```python
from build123d import *

# Parameters (mm, degrees)
TOP_EDGE_OUTLINE_W   = 86.5
TOP_EDGE_OUTLINE_H   = 39.5
TOP_EDGE_DEPTH       = 3
TOP_EDGE_DRAFT       = 45
SKETCH13_W           = 72
SKETCH13_H           = 25
DISPLAY_HOLE_DEPTH   = 6
SKETCH14_W           = 92.5
SKETCH14_H           = 45.5
SKETCH14_W_2         = 89.5
SKETCH14_H_2         = 42.5
BOSS_EXTRUDE5_DEPTH  = 5
SKETCH15_W           = 128.5
SKETCH15_H           = 45.5
SKETCH15_W_2         = 89.5
SKETCH15_H_2         = 42.5
BOSS_EXTRUDE6_DEPTH  = 2
SKETCH16_W           = 128.5
SKETCH16_H           = 45.5
SKETCH16_W_2         = 125.5
SKETCH16_H_2         = 42.5
BOSS_EXTRUDE7_DEPTH  = 37
LOFT2_OUTLINE_W      = 33
LOFT2_OUTLINE_H      = 42.5
LOFT2_DEPTH          = 1.5
LOFT2_DRAFT          = 45
SKETCH19_R           = 2.75
SKETCH19_R_2         = 2
BOSS_EXTRUDE8_DEPTH  = 1
CUT_EXTRUDE3_START   = -11
SKETCH20_R           = 2
CUT_EXTRUDE3_DEPTH   = 11
SKETCH21_W           = 12
SKETCH21_H           = 8
CUT_EXTRUDE4_DEPTH   = 11
SKETCH22_W           = 4
SKETCH22_H           = 15
BOSS_EXTRUDE9_DEPTH  = 3
SKETCH24_W           = 42.5
SKETCH24_H           = 37
CUT_EXTRUDE5_DEPTH   = 17
SKETCH26_W           = 65.330388672
SKETCH26_H           = 66.528532866
CUT_EXTRUDE6_DEPTH   = 47
SKETCH27_W           = 135.174847233
SKETCH27_H           = 89.815373094
CUT_EXTRUDE7_DEPTH   = 47
SKETCH28_W           = 107.897480511
SKETCH28_H           = 56.576939502
SKETCH28_W_2         = 83.398406197
SKETCH28_H_2         = 34.654132256
CUT_EXTRUDE9_DEPTH   = 20.5
SKETCH29_W           = 89.2
SKETCH29_H           = 42.2
SKETCH29_W_2         = 86.2
SKETCH29_H_2         = 39.2
BOSS_EXTRUDE11_DEPTH = 5


# Read off the part's stored shape, not the designer's step: Top Edge, Loft2
with BuildPart() as part:
    # Top Edge outline → Top Edge (with draft: the straight prism first)
    with BuildSketch(Plane(origin=(0, 0, 0), x_dir=(1, 0, 0), z_dir=(0, 1, 0))):
        with Locations((0.25, -0.25)):
            Rectangle(TOP_EDGE_OUTLINE_W, TOP_EDGE_OUTLINE_H)
    extrude(amount=-TOP_EDGE_DEPTH)
    # Top Edge: the draft: its side faces are tilted about the plane it starts from
    top_edge_sides = [part.faces().sort_by_distance(p)[0] for p in [
        (-43, -1.5, 0.25),
        (0.25, -1.5, 20),
        (43.5, -1.5, 0.25),
        (0.25, -1.5, -19.5),
    ]]
    draft(top_edge_sides, Plane(origin=(0, 0, 0), x_dir=(1, 0, 0), z_dir=(0, 1, 0)), TOP_EDGE_DRAFT)

    # Sketch13 → Display Hole (cut)
    with BuildSketch(Plane(origin=(0, 0, 0), x_dir=(1, 0, 0), z_dir=(0, 1, 0))):
        Rectangle(SKETCH13_W, SKETCH13_H)
    extrude(amount=-DISPLAY_HOLE_DEPTH, mode=Mode.SUBTRACT)

    # Sketch14 → Boss-Extrude5 (add)
    with BuildSketch(Plane.XZ.offset(3)):
        with Locations((0.25, 0.25)):
            Rectangle(SKETCH14_W, SKETCH14_H)
        with Locations((0.25, 0.25)):
            Rectangle(SKETCH14_W_2, SKETCH14_H_2, mode=Mode.SUBTRACT)
    extrude(amount=BOSS_EXTRUDE5_DEPTH)

    # Sketch15 → Boss-Extrude6 (add)
    with BuildSketch(Plane.XZ.offset(8)):
        with Locations((18.25, 0.25)):
            Rectangle(SKETCH15_W, SKETCH15_H)
        with Locations((0.25, 0.25)):
            Rectangle(SKETCH15_W_2, SKETCH15_H_2, mode=Mode.SUBTRACT)
    extrude(amount=BOSS_EXTRUDE6_DEPTH)

    # Sketch16 → Boss-Extrude7 (add)
    with BuildSketch(Plane.XZ.offset(10)):
        with Locations((18.25, 0.25)):
            Rectangle(SKETCH16_W, SKETCH16_H)
        with Locations((18.25, 0.25)):
            Rectangle(SKETCH16_W_2, SKETCH16_H_2, mode=Mode.SUBTRACT)
    extrude(amount=BOSS_EXTRUDE7_DEPTH)


with BuildPart() as loft2_tool:
    # Loft2 outline → Loft2 (with draft: the straight prism first)
    with BuildSketch(Plane(origin=(0, -6.5, 0), x_dir=(1, 0, 0), z_dir=(0, 1, 0))):
        with Locations((64.5, -0.25)):
            Rectangle(LOFT2_OUTLINE_W, LOFT2_OUTLINE_H)
    extrude(amount=-LOFT2_DEPTH)
    # Loft2: the draft: its side faces are tilted about the plane it starts from
    loft2_sides = [loft2_tool.faces().sort_by_distance(p)[0] for p in [
        (81, -7.25, 0.25),
        (64.5, -7.25, -21),
        (48, -7.25, 0.25),
        (64.5, -7.25, 21.5),
    ]]
    draft(loft2_sides, Plane(origin=(0, -6.5, 0), x_dir=(1, 0, 0), z_dir=(0, 1, 0)), LOFT2_DRAFT)


with BuildPart() as part_1:
    add(part.part)

    # Loft2: add loft2_tool
    add(loft2_tool.part)

    # Sketch19 → Boss-Extrude8 (add)
    with BuildSketch(Plane(origin=(0, -6.5, 0), x_dir=(1, 0, 0), z_dir=(0, 1, 0))):
        with Locations(Location((64.5, 3, 0), (0, 0, 270))):
            Circle(SKETCH19_R)
        with Locations(Location((64.5, 3, 0), (0, 0, 270))):
            Circle(SKETCH19_R_2, mode=Mode.SUBTRACT)
    extrude(amount=BOSS_EXTRUDE8_DEPTH)

    # Sketch20 → Cut-Extrude3 (cut)
    with BuildSketch(Plane(origin=(0, -6.5, 0), x_dir=(1, 0, 0), z_dir=(0, 1, 0)).offset(CUT_EXTRUDE3_START)):
        with Locations(Location((64.5, 3, 0), (0, 0, 90))):
            Circle(SKETCH20_R)
    extrude(amount=CUT_EXTRUDE3_DEPTH, mode=Mode.SUBTRACT)

    # Sketch21 → Cut-Extrude4 (cut)
    with BuildSketch(Plane(origin=(82.5, 0, 0), x_dir=(0, 0, -1), z_dir=(1, 0, 0))):
        with Locations((0, -43)):
            Rectangle(SKETCH21_W, SKETCH21_H)
    extrude(amount=-CUT_EXTRUDE4_DEPTH, mode=Mode.SUBTRACT)

    # Sketch22 → Boss-Extrude9 (add)
    with BuildSketch(Plane.XZ.offset(3)):
        with Locations((-38, 0)):
            Rectangle(SKETCH22_W, SKETCH22_H)
    extrude(amount=BOSS_EXTRUDE9_DEPTH)

    # Sketch24 → Cut-Extrude5 (cut)
    with BuildSketch(Plane.ZY.offset(-81)):
        with Locations((0.25, -28.5)):
            Rectangle(SKETCH24_W, SKETCH24_H)
    extrude(amount=-CUT_EXTRUDE5_DEPTH, mode=Mode.SUBTRACT)

    # Sketch26 → Cut-Extrude6 (cut)
    with BuildSketch(Plane(origin=(46.5, 0, 0), x_dir=(0, 0, -1), z_dir=(1, 0, 0))):
        with Locations((4.479516554, -23.405372169)):
            Rectangle(SKETCH26_W, SKETCH26_H)
    extrude(amount=CUT_EXTRUDE6_DEPTH, mode=Mode.SUBTRACT)

    # Sketch27 → Cut-Extrude7 (cut)
    with BuildSketch(Plane.XZ.offset(10)):
        with Locations((-2.496201378, -4.177518392)):
            Rectangle(SKETCH27_W, SKETCH27_H)
    extrude(amount=CUT_EXTRUDE7_DEPTH, mode=Mode.SUBTRACT)

    # Sketch28 → Cut-Extrude9 (cut)
    with BuildSketch(Plane.XZ.offset(3)):
        with Locations((0.925246346, -0.196985684)):
            Rectangle(SKETCH28_W, SKETCH28_H)
        with Locations((-0.40760533, 0.012173471)):
            Rectangle(SKETCH28_W_2, SKETCH28_H_2, mode=Mode.SUBTRACT)
    extrude(amount=CUT_EXTRUDE9_DEPTH, mode=Mode.SUBTRACT)

    # Sketch29 → Boss-Extrude11 (add)
    with BuildSketch(Plane.XZ.offset(3)):
        with Locations((0.25, 0.25)):
            Rectangle(SKETCH29_W, SKETCH29_H)
        with Locations((0.25, 0.25)):
            Rectangle(SKETCH29_W_2, SKETCH29_H_2, mode=Mode.SUBTRACT)
    extrude(amount=BOSS_EXTRUDE11_DEPTH)


solid = part_1.part
```
The model under review builds one solid part; all positions refer to its coordinate system, in mm. A direction names the side the tool comes from. Round coordinates to 2 decimals unless told otherwise and drop trailing zeros. Loops run counter-clockwise (first coordinate to the right, second up) from the corner with the lowest first, then second, coordinate; pieces in that order, holes last.
Item 1: Take a section at A-A (y = -5). Write out the cut boundary in (x, z), then the cut area to 3 significant figures.
Determined:
outline: (-44.35, -20.85) - (44.85, -20.85) - (44.85, 21.35) - (-44.35, 21.35) - close; (-40, -7.5) - (-36, -7.5) - (-36, 7.5) - (-40, 7.5) - close; hole (-42.85, -19.35) - (43.35, -19.35) - (43.35, 19.85) - (-42.85, 19.85) - close
area: 445 mm2
Item 2: Take a section at D-D (z = 11). Write out the cut boundary in (x, y), then the cut area to 3 significant figures.
Determined:
outline: (-46, -3) - (-44.35, -3) - (-44.35, -8) - (-42.85, -8) - (-42.85, -3) - (-36, -3) - (-36, 0) - (-43, 0) - close; (36, -3) - (43.35, -3) - (43.35, -8) - (44.85, -8) - (44.85, -3) - (46.5, -3) - (43.5, 0) - (36, 0) - close
area: 67.5 mm2
Item 3: Take a section at B-B (x = 30). Write out the cut boundary in (y, z), then the cut area to 3 significant figures.
Determined:
outline: (-8, -20.85) - (-3, -20.85) - (-3, -22.5) - (0, -19.5) - (0, -12.5) - (-3, -12.5) - (-3, -19.35) - (-8, -19.35) - close; (-8, 19.85) - (-3, 19.85) - (-3, 12.5) - (0, 12.5) - (0, 20) - (-3, 23) - (-3, 21.35) - (-8, 21.35) - close
area: 67.5 mm2
Item 4: Mouldability with a two-part tool opening along Z and no side actions: class faces 1 (the face through (0, -3, 14)), 2 (the face through (0, -1, 21)), 3 (the face through (45, -1.5, 0.6)) as released by +Z, released by -Z, zero draft, split by the parting line, or undercut.
Determined:
face 1: undercut
face 2: released by +Z
face 3: zero draft
Item 5: Take a section at C-C (z = -5). Write out the cut boundary in (x, y).
Determined:
outline: (-46, -3) - (-44.35, -3) - (-44.35, -8) - (-42.85, -8) - (-42.85, -3) - (-40, -3) - (-40, -6) - (-36, -6) - (-36, 0) - (-43, 0) - close; (36, -3) - (43.35, -3) - (43.35, -8) - (44.85, -8) - (44.85, -3) - (46.5, -3) - (43.5, 0) - (36, 0) - close
Item 6: For faces 4 (the face through (-42.85, -5, 0)), 5 (the face through (-1, -1, 12.5)), 6 (the face through (0, -5, 21.35)), list the 3-axis set-ups (+Z, -Z, +X, -X, +Y, -Y) from which the entire face can be reached by the end or side of a thin tool; tool diameter is ignored.
Determined:
face 4: -Y
face 5: +Y, -Y
face 6: +Z, +X, -X, -Y
Item 7: For line 1 (Z direction, x = 13, y = -3.25); line 2 (X direction, y = -7, z = 6.5); line 3 (Y direction, x = 38.5, z = 12.5), list the stretches that pass through material, from the lowest coordinate up.
Determined:
line 1: z = -20.85 to -19.35, 19.85 to 21.35
line 2: x = -44.35 to -42.85, 43.35 to 44.85
line 3: y = -3 to 0
Item 8: Clearance check with flat-ended pins moving along their axes: pin 1 Ø2.5 at (y, z) = (-5.5, 8.5) entering from +X; pin 2 Ø4 at (y, z) = (-6.5, -2.5) entering from -X; pin 3 Ø1.8 at (y, z) = (-1.5, 1.5) entering from +X. State where each tip first meets the part, or that it passes through.
Determined:
pin 1: stops at x = 44.85
pin 2: stops at x = -44.35
pin 3: stops at x = 45.9
